from build123d import *

# Parameters (mm, degrees)
SKETCH1_R           = 1.5
BOSS_EXTRUDE1_DEPTH = 2
BOSS_EXTRUDE2_START = 2
SKETCH1_3_W         = 4.666904756
SKETCH1_3_H         = 4.666904756
BOSS_EXTRUDE2_DEPTH = 40
SKETCH3_R           = 2.15
CUT_EXTRUDE1_DEPTH  = 2.25


with BuildPart() as part:
    # Sketch1 → Boss-Extrude1 (new body)
    with BuildSketch(Plane(origin=(0, 0, 0), x_dir=(0, 0, -1), z_dir=(1, 0, 0))):
        with BuildLine():
            Line((-19.86340857, -2.333452378), (19.86340857, -2.333452378))
            ThreePointArc((19.86340857, -2.333452378), (0, 20), (-19.86340857, -2.333452378))
        make_face()
        with Locations((-14.75, 0)):
            Circle(SKETCH1_R, mode=Mode.SUBTRACT)
        with Locations((14.75, 0)):
            Circle(SKETCH1_R, mode=Mode.SUBTRACT)
        with Locations((-8.485281374, 8.485281374)):
            Circle(SKETCH1_R, mode=Mode.SUBTRACT)
        with Locations((8.485281374, 8.485281374)):
            Circle(SKETCH1_R, mode=Mode.SUBTRACT)
        with Locations((0, 14.75)):
            Circle(SKETCH1_R, mode=Mode.SUBTRACT)
    extrude(amount=BOSS_EXTRUDE1_DEPTH)

    # Sketch1<3> → Boss-Extrude2 (add)
    with BuildSketch(Plane(origin=(0, 0, 0), x_dir=(0, 0, -1), z_dir=(1, 0, 0)).offset(BOSS_EXTRUDE2_START)):
        Rectangle(SKETCH1_3_W, SKETCH1_3_H)
        with BuildLine():
            Line((2.333452378, 2.333452378), (2.333452378, -2.333452378))
            ThreePointArc((2.333452378, -2.333452378), (3.048802457, -1.262855327), (3.3, 0))
            ThreePointArc((3.3, 0), (3.048802457, 1.262855327), (2.333452378, 2.333452378))
        make_face()
        with BuildLine():
            ThreePointArc((2.333452378, 2.333452378), (0, 3.3), (-2.333452378, 2.333452378))
            Line((-2.333452378, 2.333452378), (2.333452378, 2.333452378))
        make_face()
        with BuildLine():
            ThreePointArc((-2.333452378, 2.333452378), (-3.3, 0), (-2.333452378, -2.333452378))
            Line((-2.333452378, -2.333452378), (-2.333452378, 2.333452378))
        make_face()
    extrude(amount=BOSS_EXTRUDE2_DEPTH)

    # Sketch3 → Cut-Extrude1 (cut)
    with BuildSketch(Plane(origin=(42, 0, 0), x_dir=(0, 0, -1), z_dir=(1, 0, 0))):
        Circle(SKETCH3_R)
    extrude(amount=-CUT_EXTRUDE1_DEPTH, mode=Mode.SUBTRACT)


solid = part.part
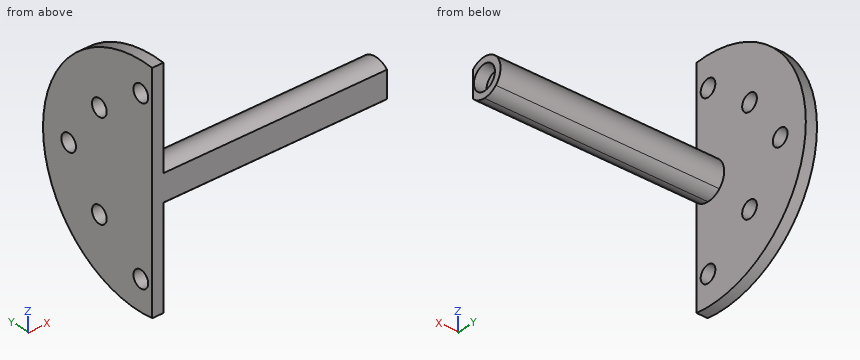
The listing builds one solid part. Answer for the finished solid, in the listing's coordinates (mm). Give positions to 0.01 mm unless a question says otherwise; leave off trailing zeros. Loops run counter-clockwise (first coordinate to the right, second up) from the corner with the lowest first, then second, coordinate; pieces in that order, holes last.
Item 1: Find the intervals of material crossed by line 1 along Y through (x, z) = (9, 0); line 2 along X through (y, z) = (-0.75, -11.5); line 3 along X through (y, z) = (1, -1.5), in increasing order.
Derived:
line 1: y = -2.33 to 3.3
line 2: x = 0 to 2
line 3: x = 0 to 39.75
Item 2: A cutting plane is placed at A-A (z = -14.75). Give the vertices of the cut face in (x, y), then the cut area to 3 significant figures.
Derived:
outline: (0, -2.33) - (2, -2.33) - (2, -1.5) - (0, -1.5) - close; (0, 1.5) - (2, 1.5) - (2, 13.51) - (0, 13.51) - close
area: 25.7 mm2
Item 3: A cutting plane is placed at C-C (x = 17.5). Give the vertices of the cut face in (y, z).
Derived:
outline: (-2.33, -2.33) arc R3.3 ccw (long way) to (-2.33, 2.33) - close
Item 4: Each of these flat-tipped pins is pushed along its axis until it touches: pin 1 Ø1.8 at (y, z) = (8.49, 8.49) entering from +X; pin 2 Ø5 at (x, z) = (33, -3) entering from +Y; pin 3 Ø8 at (x, y) = (35.5, 4.5) entering from -Z; pin 4 Ø6 at (y, z) = (1, 7) entering from +X. Where does it stop, or does it pass through?
Derived:
pin 1: passes through
pin 2: stops at y = 3.26
pin 3: stops at z = -3.26
pin 4: stops at x = 2
Item 5: A cutting plane is placed at D-D (y = 11.5). Give the vertices of the cut face in (x, z).
Derived:
outline: (0, -16.36) - (2, -16.36) - (2, 16.36) - (0, 16.36) - close
Item 6: A cutting plane is placed at B-B (y = 14.75). Give the vertices of the cut face in (x, z), then the cut area to 3 significant figures.
Derived:
outline: (0, -13.51) - (2, -13.51) - (2, -1.5) - (0, -1.5) - close; (0, 1.5) - (2, 1.5) - (2, 13.51) - (0, 13.51) - close
area: 48.0 mm2
